Read the model definition and answer for the solid it produces. Units are mm, in the model's axes. Face numbers are marked on the shaded views. Coordinates: 2 decimals unless noted, no trailing zeros. Order: outer loops, then holes, each group sorted by start corner. A loop starts at its lowest first (then second) coordinate and runs counter-clockwise, first axis right, second up. Notation, with made-up numbers: (72.25, 16) -> (96.25, 16) arc R24 cw to (96.25, 49) -> close; hole circle Ø10 at (4, -23.5). An arc over 180 degrees is marked (long way). Use CSV: the item, a comma, the result in double quotes.
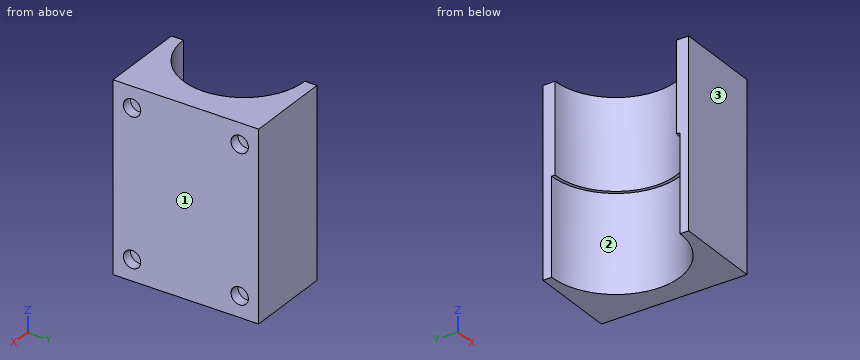
```python
from build123d import *

# Parameters (mm, degrees)
SKETCH1_W           = 25
SKETCH1_H           = 42
BOSS_EXTRUDE1_DEPTH = 54
CUT_EXTRUDE1_START  = -28
SKETCH2_R           = 18.5
CUT_EXTRUDE1_DEPTH  = 28
CUT_EXTRUDE2_REACH  = 64.714
SKETCH3_R           = 17.5
SKETCH4_R           = 2.5
CUT_EXTRUDE3_DEPTH  = 3


with BuildPart() as part:
    # Sketch1 → Boss-Extrude1 (new body)
    with BuildSketch(Plane.XY):
        with Locations((11.5, 0)):
            Rectangle(SKETCH1_W, SKETCH1_H)
    extrude(amount=-BOSS_EXTRUDE1_DEPTH)

    # Sketch2 → Cut-Extrude1 (cut)
    with BuildSketch(Plane(origin=(0, 0, -54), x_dir=(-1, 0, 0), z_dir=(0, 0, -1)).offset(CUT_EXTRUDE1_START)):
        with Locations((1, 0)):
            Circle(SKETCH2_R)
    extrude(amount=CUT_EXTRUDE1_DEPTH, mode=Mode.SUBTRACT)

    # Sketch3 → Cut-Extrude2 (cut, up to next)
    with BuildSketch(Plane.XY, mode=Mode.PRIVATE) as cut_extrude2_sk1:
        with Locations((-1, 0)):
            Circle(SKETCH3_R)
    cut_extrude2_tool1 = extrude(cut_extrude2_sk1.sketch, amount=-CUT_EXTRUDE2_REACH, mode=Mode.PRIVATE) & part.part
    add(cut_extrude2_tool1.solids().sort_by_distance((-1, 0, 0))[0], mode=Mode.SUBTRACT)

    # Sketch4 → Cut-Extrude3 (cut)
    with BuildSketch(Plane(origin=(24, 0, 0), x_dir=(0, 0, -1), z_dir=(1, 0, 0))):
        with Locations(Location((6, 15.5, 0), (0, 0, 90))):
            Circle(SKETCH4_R)
        with Locations(Location((48, 15.5, 0), (0, 0, 90))):
            Circle(SKETCH4_R)
        with Locations(Location((6, -15.5, 0), (0, 0, 90))):
            Circle(SKETCH4_R)
        with Locations(Location((48, -15.5, 0), (0, 0, 90))):
            Circle(SKETCH4_R)
    extrude(amount=-CUT_EXTRUDE3_DEPTH, mode=Mode.SUBTRACT)


solid = part.part
```
Item 1: Find section D-D, the plane x = 13.5. Give the vertices of the cut face in (y, z), then the cut area to 3 significant figures.
Return value:
outline,"(-21, -54) -> (-11.49, -54) -> (-11.49, -26) -> (-9.8, -26) -> (-9.8, 0) -> (-21, 0) -> close; (9.8, -26) -> (11.49, -26) -> (11.49, -54) -> (21, -54) -> (21, 0) -> (9.8, 0) -> close"
area,"1,120 mm^2"
Item 2: Find section C-C, the plane y = -14. Give the vertices of the cut face in (x, z).
Return value:
outline,"(9.5, -26) -> (11.09, -26) -> (11.09, -54) -> (24, -54) -> (24, -50) -> (21, -50) -> (21, -46) -> (24, -46) -> (24, -8) -> (21, -8) -> (21, -4) -> (24, -4) -> (24, 0) -> (9.5, 0) -> close"
Item 3: Find section A-A, the plane z = -6. Give the vertices of the cut face in (x, y).
Return value:
outline,"(-1, -21) -> (24, -21) -> (24, -18) -> (21, -18) -> (21, -13) -> (24, -13) -> (24, 13) -> (21, 13) -> (21, 18) -> (24, 18) -> (24, 21) -> (-1, 21) -> (-1, 17.5) arc R17.5 cw to (-1, -17.5) -> close"
Item 4: Find section B-B, the plane x = 2.5. Give the vertices of the cut face in (y, z).
Return value:
outline,"(-21, -54) -> (-18.17, -54) -> (-18.17, -26) -> (-17.15, -26) -> (-17.15, 0) -> (-21, 0) -> close; (17.15, -26) -> (18.17, -26) -> (18.17, -54) -> (21, -54) -> (21, 0) -> (17.15, 0) -> close"
Item 5: The mould has two halves that part along Y. Classify the marked faces 1, 2 and 3: +Y half, -Y half, draft (parallel to the pull), parting line (faces both ways), or undercut.
Return value:
face 1,"draft"
face 2,"undercut"
face 3,"-Y half"
Item 6: Each of these flat-tipped pins is pushed along its axis until it touches: P1, Ø1.5, axis at y = 15, z = -6.5, coming from the +X side; P2, Ø3, axis at y = -6.5, z = -38.5, coming from the -X side; P3, Ø4, axis at y = 13.5, z = -7, coming from the -X side; P4, Ø15, axis at x = 7.5, y = -2, coming from the -Z side. Where does it stop, or does it pass through?
Return value:
P1,"stops at x = 21"
P2,"stops at x = 15.68"
P3,"stops at x = 7.12"
P4,"passes through"
Item 7: Straight lines are drawn through the part: line 1 along Z through (x, y) = (21.6, 15.5); line 2 along X through (y, z) = (-0.5, -14); line 3 along Y through (x, z) = (2.75, -40.5). For each, find the intervals that lie inside material, in ascending order.
Return value:
line 1,"z = -54 to -50.5, -45.5 to -8.5, -3.5 to 0"
line 2,"x = 16.49 to 24"
line 3,"y = -21 to -18.12, 18.12 to 21"
